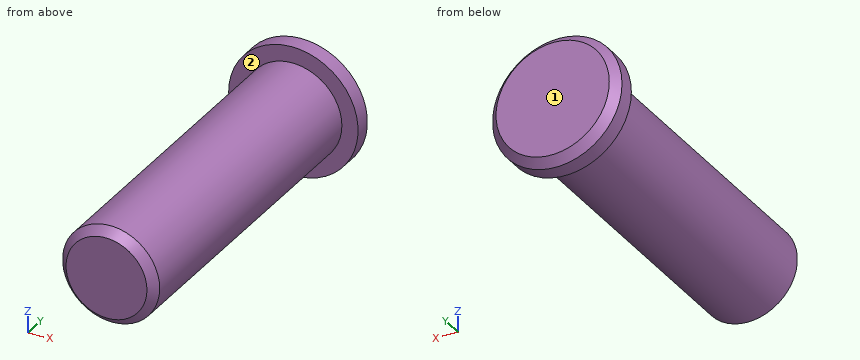
Autodesk Inventor part; units mm, degrees
ref_plane "YZ Plane" through (0, 0, 0) normal (1, 0, 0) x (0, 1, 0)
ref_plane "XZ Plane" through (0, 0, 0) normal (0, 1, 0) x (-1, 0, 0)
ref_plane "XY Plane" through (0, 0, 0) normal (0, 0, 1) x (1, 0, 0)
sketch "Sketch1" plane through (0, 0, 0) normal (0, 1, 0) x (-1, 0, 0)
  circle A0 centre (0, 0) radius 4
  dimension "d0" = 8
extrude "Extrusion1" add sketch "Sketch1" along normal blind 1.5
sketch "Sketch2" plane through (0, 0, 0) normal (0, -1, 0) x (1, 0, 0)
  circle A0 centre (0, 0) radius 3
  dimension "d4" = 6
extrude "Extrusion2" add sketch "Sketch2" along normal blind 20
chamfer "Chamfer1" distance 0.5 angle 45 1 edges at (4, 1.5, 0)
chamfer "Chamfer2" distance 0.5 angle 45 1 edges at (-3, -20, 0)
properties part number "reverse gear crankrod pin 1"
The model under review builds one solid part; all positions refer to its coordinate system, in mm. Face numbers are marked on the shaded views. A direction names the side the tool comes from. Give positions to 0.01 mm unless a question says otherwise; leave off trailing zeros. Loops run counter-clockwise (first coordinate to the right, second up) from the corner with the lowest first, then second, coordinate; pieces in that order, holes last. Notation, with made-up numbers: (-20.5, 0) -> (1.5, 0) arc R31 cw to (1.5, 24) -> close; hole circle Ø1 at (8.5, 2). An arc over 180 degrees is marked (long way). Answer as a JSON object with one key per item and string values. Group by question number.
Q1. Wall thickness on line 1 along Y through (x, z) = (1.75, -2.5); line 2 along Z through (x, y) = (-2, -13.25); line 3 along X through (y, z) = (-11, -2.25): over which ranges is each line inside the solid? List them lowest first.
Q2. Tool access review of the marked faces 1 and 2: name each direction out of +Z, -Z, +X, -X, +Y, -Y from which nothing blocks a thin tool from reaching the whole face with its end or side.
Q3. Take a section at A-A (x = 0). Write out the cut boundary in (y, z).
Q4. Insertion check: pin 1 (3 mm diameter, centred on x = 1.5, y = -14, fed in from -Z); pin 2 (1.5 mm diameter, centred on x = -2.5, y = -6.5, fed in from -Z). Each pin has a flat end and moves straight along its axis. Give the tip position at first contact, or say it passes through.
Q5. Take a section at B-B (z = 0). Write out the cut boundary in (x, y).
Q6. Take a section at C-C (y = -0.75). Write out the cut boundary in (x, z), plus the area to 3 significant figures.
Answer below:
{
 "1": {"line 1": "y = 0 to 1.5", "line 2": "z = -2.24 to 2.24", "line 3": "x = -1.98 to 1.98"},
 "2": {"face 1": "+Z, -Z, +X, -X, +Y", "face 2": "-Y"},
 "3": {"outline": "(-20, -2.5) -> (-19.5, -3) -> (0, -3) -> (0, -4) -> (1, -4) -> (1.5, -3.5) -> (1.5, 3.5) -> (1, 4) -> (0, 4) -> (0, 3) -> (-19.5, 3) -> (-20, 2.5) -> close"},
 "4": {"pin 1": "stops at z = -3", "pin 2": "stops at z = -2.44"},
 "5": {"outline": "(-4, 0) -> (-3, 0) -> (-3, -19.5) -> (-2.5, -20) -> (2.5, -20) -> (3, -19.5) -> (3, 0) -> (4, 0) -> (4, 1) -> (3.5, 1.5) -> (-3.5, 1.5) -> (-4, 1) -> close"},
 "6": {"outline": "circle Ø6 at (0, 0)", "area": "28.3 mm2"}
}
